```python
from build123d import *

# Parameters (mm, degrees)
F1_DEPTH = 152.4


# Not quite as in the source:
# - ends of sketch curves that miss each other by under 0.0002 mm in the source are joined


with BuildPart() as f1:
    # F0 (on Front) → F1 (new body)
    with BuildSketch(Plane.XZ):
        with BuildLine():
            ThreePointArc((-6.352921, 3.1764732), (-8.2136484806, 7.6686667194), (-12.705842, 9.5293942))
            ThreePointArc((-12.705842, 9.5293942), (-17.1980355194, 7.6686667194), (-19.058763, 3.1764732))
            Line((-19.058763, 3.1764732), (-14.2940786, 3.1764732))
            Line((-14.2940786, 3.1764732), (-14.2940786, -3.1764478))
            Line((-14.2940786, -3.1764478), (-7.9411576, -9.5293942))
            Line((-7.9411576, -9.5293942), (19.058763, -9.5293942))
            Line((19.058763, -9.5293942), (19.058763, -6.352921))
            ThreePointArc((19.058763, -6.352921), (16.81265726, -5.42255354), (15.8822898, -3.1764478))
            Line((15.8822898, -3.1764478), (12.705842, -3.1764478))
            ThreePointArc((12.705842, -3.1764478), (11.77549994, -5.42255354), (9.5293942, -6.352921))
            ThreePointArc((9.5293942, -6.352921), (1.7744943071, -3.4575238304), (-3.1764521069, 3.1764716036))
            Line((-3.1764521069, 3.1764716036), (-6.352921, 3.1764732))
        make_face()
    extrude(amount=F1_DEPTH)


solid = f1.part
```
Source: CAD feature listing. Evaluate the final solid. Frame: model axes, mm. A direction names the side the tool comes from. Give positions to 0.01 mm unless a question says otherwise; leave off trailing zeros. Write each loop counter-clockwise with the first axis right and the second up, starting at its lowest first coordinate (ties: lowest second). Pieces come first, ordered by that corner, then holes.
1. Section query D-D (z = 8). Return the cut outline in (x, y).
2. First-contact query: pin 1 (4 mm diameter, centred on x = -17, y = -59, fed in from -Z); pin 2 (1 mm diameter, centred on x = -11, y = -85, fed in from -Z); pin 3 (2 mm diameter, centred on x = -3.5, y = -32, fed in from +Z). Flat tips, straight axial feed; report the tip coordinate or a pass-through.
3. Section query A-A (z = -5). Return the cut outline in (x, y), then the cut area to 3 significant figures.
4. Access query for faces 1 (the face through (14, -75, -3.176)), 2 (the face through (-5, -152.4, -2)), 3 (the face through (1.87, -75.13, -3.53)), 4 (the face through (-17, -75, 3.176)), 5 (the face through (-5, 0, -2)). Directions: +Z, -Z, +X, -X, +Y, -Y. A direction counts if a zero-diameter tool reaches every point of the face in a straight line with its end or side. Return the directions, or none.
5. Pull-direction query (X, two-part tool) for faces 6 (the face through (-11.16, -75.13, -6.31)), 7 (the face through (19.059, -75, -8)), 8 (the face through (-5, -75, 3.176)), 9 (the face through (11.8, -75.1, -5.4)); classes: +X half, -X half, draft (parallel to the pull), parting line (faces both ways), or undercut.
6. Section query C-C (x = -5). Return the cut outline in (y, z).
7. Material intervals for line 1 along Z through (x, y) = (13.5, -136.5); line 2 along X through (y, z) = (-130, -3.75); line 3 along Z through (x, y) = (-15, -6.5), sorted ascending.
8. Section query B-B (y = -135.5). Return the cut outline in (x, z), then the cut area to 3 significant figures.
Output values:
1. outline: (-16.84, -152.4) - (-8.57, -152.4) - (-8.57, 0) - (-16.84, 0) - close
2. pin 1: stops at z = 3.18
2. pin 2: stops at z = -6.97
2. pin 3: stops at z = 3.18
3. outline: (-12.47, -152.4) - (4.34, -152.4) - (4.34, 0) - (-12.47, 0) - close; (12.13, -152.4) - (16.46, -152.4) - (16.46, 0) - (12.13, 0) - close
3. area: 3,220 mm2
4. face 1: +Z, +X, +Y, -Y
4. face 2: +Z, -Z, +X, -X, -Y
4. face 3: +Z, +Y, -Y
4. face 4: -Z, -X, +Y, -Y
4. face 5: +Z, -Z, +X, -X, +Y
5. face 6: -X half
5. face 7: +X half
5. face 8: draft
5. face 9: undercut
6. outline: (-152.4, -9.53) - (0, -9.53) - (0, 3.18) - (-152.4, 3.18) - close
7. line 1: z = -9.53 to -3.18
7. line 2: x = -13.72 to 2.18, 12.65 to 15.93
7. line 3: z = 3.18 to 9.1
8. outline: (-19.06, 3.18) - (-14.29, 3.18) - (-14.29, -3.18) - (-7.94, -9.53) - (19.06, -9.53) - (19.06, -6.35) arc R3.18 cw to (15.88, -3.18) - (12.71, -3.18) arc R3.18 cw to (9.53, -6.35) arc R14.66 cw to (-3.18, 3.18) - (-6.35, 3.18) arc R6.35 ccw to start
8. area: 305 mm2
